from build123d import *

# Parameters (mm, degrees)
CYLINDER011024_R               = 1.8
CYLINDER011024_DEPTH           = 20
CYLINDER011020_R               = 3
CYLINDER011020_DEPTH           = 20
CYLINDER011027_R               = 2
CYLINDER011027_DEPTH           = 20
CYLINDER011022_R               = 8
CYLINDER011022_DEPTH           = 10
CYLINDER011023_W               = 11
CYLINDER011023_H               = 10
CYLINDER011023_ANGLE           = 240
CYLINDER011023_PLACEMENT_ANGLE = 150
PAD001_DEPTH                   = 10


with BuildPart() as bolt_hole004:
    # Cylinder011024 → Cylinder011024 (new body)
    with BuildSketch(Plane(origin=(-1, 14, 5), x_dir=(0, 0, -1), z_dir=(1, 0, 0))):
        Circle(CYLINDER011024_R)
    extrude(amount=CYLINDER011024_DEPTH)


with BuildPart() as bolt_head_hole001:
    # Cylinder011020 → Cylinder011020 (new body)
    with BuildSketch(Plane(origin=(11.5, 14, 5), x_dir=(0, 0, -1), z_dir=(1, 0, 0))):
        Circle(CYLINDER011020_R)
    extrude(amount=CYLINDER011020_DEPTH)


with BuildPart() as obj1:
    # Cylinder011027 → Cylinder011027 (new body)
    with BuildSketch(Plane(origin=(-22, 14, 5), x_dir=(0, 0, -1), z_dir=(1, 0, 0))):
        Circle(CYLINDER011027_R)
    extrude(amount=CYLINDER011027_DEPTH)

    # Fusion009: union bolt hole004, bolt head hole001
    add(bolt_hole004.part)
    add(bolt_head_hole001.part)


with BuildPart() as cylinder011022:
    # Cylinder011022 → Cylinder011022 (new body)
    with BuildSketch(Plane.XY):
        Circle(CYLINDER011022_R)
    extrude(amount=CYLINDER011022_DEPTH)


with BuildPart() as cut023015009018:
    # Cylinder011023 → Cylinder011023 (revolve)
    with BuildSketch(Plane.XZ):
        with Locations((5.5, 5)):
            Rectangle(CYLINDER011023_W, CYLINDER011023_H)
    revolve(axis=Axis((0, 0, 0), (0, 0, 1)), revolution_arc=CYLINDER011023_ANGLE)


with BuildPart() as cut023015009018_1:
    # Cylinder011023 placement: moved
    add(cut023015009018.part.rotate(Axis((0, 0, 0), (0, 0, 1)), CYLINDER011023_PLACEMENT_ANGLE))

    # Cut023015009018: cut Cylinder011022
    add(cylinder011022.part, mode=Mode.SUBTRACT)


with BuildPart() as shaft_attachment_cut001:
    # Sketch004 → Pad001 (new body)
    with BuildSketch(Plane.XY):
        with BuildLine():
            Line((12, -2.57721), (12, 19.017869))
            ThreePointArc((12, 19.017869), (11.523224, 20.168908), (10.372186, 20.645684))
            Line((10.372186, 20.645684), (9.627814, 20.645684))
            ThreePointArc((9.627814, 20.645684), (8.476776, 20.168908), (8, 19.017869))
            Line((8, 19.017869), (8, 0))
            ThreePointArc((-8, 0), (0, -8), (8, 0))
            Line((-8, 0), (-8, 18.544726))
            ThreePointArc((-8, 18.544726), (-8.476776, 19.695765), (-9.627814, 20.17254))
            Line((-9.627814, 20.17254), (-13.372186, 20.17254))
            ThreePointArc((-13.372186, 20.17254), (-14.523224, 19.695765), (-15, 18.544726))
            Line((-15, 18.544726), (-15, -2.57721))
            ThreePointArc((-15, -2.57721), (-1.5, -16.07721), (12, -2.57721))
        make_face()
    extrude(amount=PAD001_DEPTH)

    # Fusion008: union Cut023015009018
    add(cut023015009018_1.part)

    # Cut023015009017: cut obj1
    add(obj1.part, mode=Mode.SUBTRACT)


with BuildPart() as part_mirroring003:
    # Part__Mirroring003: instance of shaft attachment  cut001
    add(shaft_attachment_cut001.part.mirror(Plane(origin=(0, -50, 0), x_dir=(1, 0, 0), z_dir=(0, 1, 0))))


solid = part_mirroring003.part
Work out the finished part from the listing and answer in its coordinate system (mm). A direction names the side the tool comes from. Round coordinates to 2 decimals unless told otherwise and drop trailing zeros. Write each loop counter-clockwise with the first axis right and the second up, starting at its lowest first coordinate (ties: lowest second). Pieces come first, ordered by that corner, then holes.
1) The mould has two halves that part along Z. Classify faces 4 (the cylindrical face through (-1.797, -83.926, 4.93)), 5 (the flat face through (-8, -103, 0)), 6 (the cylindrical face through (-11.549, -115.686, 3.925)): pulls with the +Z half, pulls with the -Z half, needs draft (parallel to the pull), parting line crosses it, or undercut.
2) A tool of negligible diameter and unlimited length cuts with its end or side. For faces 1 (the cylindrical face through (11.746, -116.974, 5.391)), 2 (the flat face through (-11, -120.173, 5)), 3 (the flat face through (7.457, -104.305, 5.07)), from which of +Z, -Z, +X, -X, +Y, -Y can it reach the whole face along a straight path? Write none if from no direction.
3) Given pin 1 Ø8 at (x, y) = (-10, -105) entering from -Z; pin 2 Ø4 at (x, z) = (-11.5, 4) entering from -Y; pin 3 Ø1.8 at (y, z) = (-112.5, 4.5) entering from +X; pin 4 Ø1 at (x, z) = (8.5, 8.5) entering from -Y, each flat-ended and moving along its own axis, determine where each tip first touches the part or whether it passes through.
4) A cutting plane is placed at A-A (y = -106). Give the vertices of the cut face in (x, z).
5) A cutting plane is placed at D-D (y = -99). Give the vertices of the cut face in (x, z), plus the area to 3 significant figures.
6) Straight lines are drawn through the part: line 1 (X direction, y = -118, z = 1.25); line 2 (Z direction, x = 11.7, y = -114); line 3 (Z direction, x = 8.75, y = -114). For each, find the intervals that lie inside material, in ascending order.
7) A cutting plane is placed at C-C (x = -8.5). Give the vertices of the cut face in (y, z).
Completed:
1. face 4: needs draft
1. face 5: pulls with the -Z half
1. face 6: undercut
2. face 1: +X
2. face 2: +Z, -Z, -X, -Y
2. face 3: +Z, -Z, -Y
3. pin 1: stops at z = 0
3. pin 2: stops at y = -120.17
3. pin 3: stops at x = 11.5
3. pin 4: stops at y = -120.52
4. outline: (-15, 0) - (-8, 0) - (-8, 10) - (-15, 10) - close; (8, 0) - (12, 0) - (12, 10) - (8, 10) - close
5. outline: (-15, 0) - (-7.94, 0) - (-7.94, 10) - (-15, 10) - close; (7.94, 0) - (12, 0) - (12, 10) - (7.94, 10) - close
5. area: 111 mm2
6. line 1: x = -15 to -8, 8 to 12
6. line 2: z = 0 to 2, 8 to 10
6. line 3: z = 0 to 3.2, 6.8 to 10
7. outline: (-119.72, 0) - (-85.88, 0) - (-85.88, 10) - (-119.72, 10) - close; hole circle Ø4 at (-114, 5)
